The drawing under review shows one solid part. Ordinate dimensions are in mm from its lowest x, y, z. A direction names the side the tool comes from. Coordinates: 2 decimals unless noted, no trailing zeros. Order: outer loops, then holes, each group sorted by start corner. A loop starts at its lowest first (then second) coordinate and runs counter-clockwise, first axis right, second up.
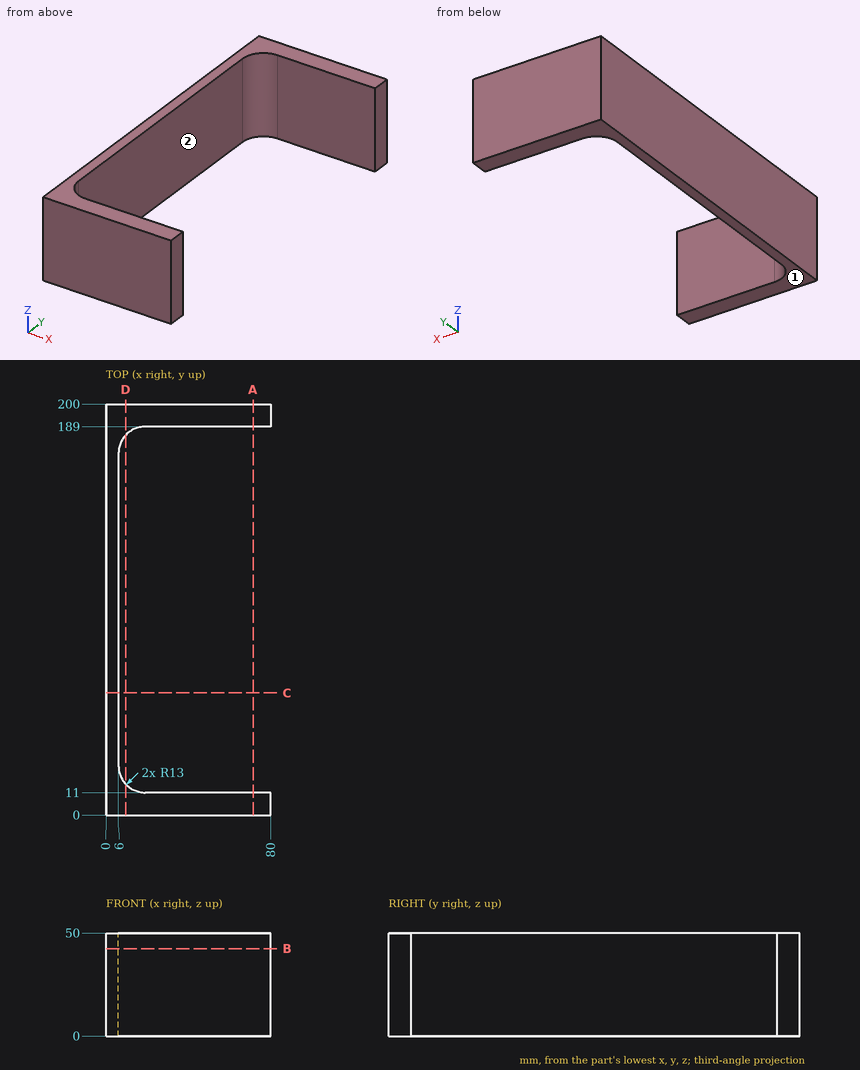
(1) Consider section C-C (y = 59.5). Give the boundary of the cut face in (x, z).
(2) Tool access review of the marked faces 1 and 2: name each direction out of +Z, -Z, +X, -X, +Y, -Y from which nothing blocks a thin tool from reaching the whole face with its end or side.
(3) Consider section A-A (x = 71.5). Give the boundary of the cut face in (y, z), then the cut area to 3 significant figures.
(4) Insertion check: pin 1 Ø3 at (y, z) = (51, 12.5) entering from -X; pin 2 Ø15 at (y, z) = (95, 24) entering from +X. Each pin has a flat end and moves straight along its axis. Give the tip position at first contact, or say it passes through.
(5) Consider section B-B (z = 42.5). Give the boundary of the cut face in (x, y), then the cut area to 3 significant figures.
(6) Consider section D-D (x = 9.5). Give the boundary of the cut face in (y, z), then the cut area to 3 significant figures.
(7) Wall thickness on line 1 (Y direction, x = 34.5, z = 5); line 2 (X direction, y = 139.5, z = 31.5); line 3 (Y direction, x = 14.5, z = 26): over which ranges is each line inside the solid? List them lowest first.
Findings:
1. outline: (0, 0) - (6, 0) - (6, 50) - (0, 50) - close
2. face 1: -Z, +X, -X, +Y, -Y
2. face 2: +Z, -Z, +X
3. outline: (0, 0) - (11, 0) - (11, 50) - (0, 50) - close; (189, 0) - (200, 0) - (200, 50) - (189, 50) - close
3. area: 1,100 mm2
4. pin 1: stops at x = 0
4. pin 2: stops at x = 6
5. outline: (0, 0) - (80, 0) - (80, 11) - (19, 11) arc R13 cw to (6, 24) - (6, 176) arc R13 cw to (19, 189) - (80, 189) - (80, 200) - (0, 200) - close
5. area: 2,900 mm2
6. outline: (0, 0) - (15.13, 0) - (15.13, 50) - (0, 50) - close; (184.87, 0) - (200, 0) - (200, 50) - (184.87, 50) - close
6. area: 1,510 mm2
7. line 1: y = 0 to 11, 189 to 200
7. line 2: x = 0 to 6
7. line 3: y = 0 to 11.8, 188.2 to 200
